from build123d import *

# Parameters (mm, degrees)
SCHIZZO1_R                    = 4
ESTRUSIONE_ESTRUSIONE1_DEPTH  = 70
TAGLIO_ESTRUSIONE1_DEPTH      = 92.446705791
TAGLIO_ESTRUSIONE1_DEPTH_BACK = 92.446705791
SCHIZZO2_W                    = 54
SCHIZZO2_H                    = 49.5
SCHIZZO4_R                    = 5
TAGLIO_ESTRUSIONE2_DEPTH      = 92.446705791


with BuildPart() as part:
    # Schizzo1 → Estrusione-Estrusione1 (new body)
    with BuildSketch(Plane.XY):
        with BuildLine():
            Line((-12.5, 0), (12.5, 0))
            Line((12.5, 0), (12.5, 45))
            ThreePointArc((12.5, 45), (0, 57.5), (-12.5, 45))
            Line((-12.5, 45), (-12.5, 0))
        make_face()
        with Locations((0, 45)):
            Circle(SCHIZZO1_R, mode=Mode.SUBTRACT)
    extrude(amount=ESTRUSIONE_ESTRUSIONE1_DEPTH)

    # Schizzo2 → Taglio-Estrusione1 (cut, two sides: drawn at the far end of the back side and taken through both)
    with BuildSketch(Plane(origin=(0, 0, 0), x_dir=(0, 0, -1), z_dir=(1, 0, 0)).offset(-TAGLIO_ESTRUSIONE1_DEPTH_BACK)):
        with Locations((-35, 32.75)):
            Rectangle(SCHIZZO2_W, SCHIZZO2_H)
    extrude(amount=TAGLIO_ESTRUSIONE1_DEPTH + TAGLIO_ESTRUSIONE1_DEPTH_BACK, mode=Mode.SUBTRACT)

    # Schizzo4 → Taglio-Estrusione2 (cut, through all)
    with BuildSketch(Plane.XZ):
        with Locations((0, 18)):
            Circle(SCHIZZO4_R)
        with Locations((0, 52)):
            Circle(SCHIZZO4_R)
    extrude(amount=-TAGLIO_ESTRUSIONE2_DEPTH, mode=Mode.SUBTRACT)


solid = part.part
Source: CAD feature listing. Evaluate the final solid. Frame: model axes, mm. A direction names the side the tool comes from. Round coordinates to 2 decimals unless told otherwise and drop trailing zeros. Loops run counter-clockwise (first coordinate to the right, second up) from the corner with the lowest first, then second, coordinate; pieces in that order, holes last. Notation, with made-up numbers: (20.5, 53) - (42.5, 53) arc R27 ccw to (42.5, 92) - close; hole circle Ø4 at (10.5, 44). An arc over 180 degrees is marked (long way). Write item = value, one per line. Start each with the question number.
Item 1: Section query B-B on z = 52. Output: boundary loops of the cut face in (x, y), plus the area to 3 significant figures.
Item 2: Mould query, pull axis X, two halves, no side actions, for faces 1 (the face through (-0.651, 3.944, 56.957)), 2 (the face through (12.5, 7, 35)), 3 (the face through (0, 29, 70)). Classes: released by +X, released by -X, zero draft, split by the parting line, or undercut.
Item 3: Section query C-C on x = 0. Output: boundary loops of the cut face in (y, z), plus the area to 3 significant figures.
Item 4: Reachability of faces 4 (the face through (0, 0, 35)), 5 (the face through (0, 32, 8)) from +Z, -Z, +X, -X, +Y, -Y: full face, straight path, thin tool, end or side. Return the list, or none.
Item 5: Section query A-A on y = 17. Output: boundary loops of the cut face in (x, z).
Item 6: Material intervals for line 1 (Z direction, x = 0, y = 3); line 2 (Z direction, x = -0.5, y = 32.5); line 3 (X direction, y = 45, z = 66.5), sorted ascending.
Item 7: Section query D-D on z = 39. Output: boundary loops of the cut face in (x, y).
Results list:
q1.outline = (-12.5, 0) - (-5, 0) - (-5, 8) - (-12.5, 8) - close; (5, 0) - (12.5, 0) - (12.5, 8) - (5, 8) - close
q1.area = 120 mm²
q2.face_1 = undercut
q2.face_2 = released by +X
q2.face_3 = zero draft
q3.outline = (0, 0) - (41, 0) - (41, 8) - (8, 8) - (8, 13) - (0, 13) - close; (0, 23) - (8, 23) - (8, 47) - (0, 47) - close; (0, 57) - (8, 57) - (8, 62) - (41, 62) - (41, 70) - (0, 70) - close; (49, 0) - (57.5, 0) - (57.5, 8) - (49, 8) - close; (49, 62) - (57.5, 62) - (57.5, 70) - (49, 70) - close
q3.area = 1,060 mm²
q4.face_4 = +Z, -Z, +X, -X, -Y
q4.face_5 = +X, -X, +Y
q5.outline = (-12.5, 0) - (12.5, 0) - (12.5, 8) - (-12.5, 8) - close; (-12.5, 62) - (12.5, 62) - (12.5, 70) - (-12.5, 70) - close
q6.line_1 = 0 to 13, 23 to 47, 57 to 70
q6.line_2 = 0 to 8, 62 to 70
q6.line_3 = -12.5 to -4, 4 to 12.5
q7.outline = (-12.5, 0) - (12.5, 0) - (12.5, 8) - (-12.5, 8) - close
